The drawing under review shows one solid part. Ordinate dimensions are in mm from its lowest x, y, z. Coordinates: 2 decimals unless noted, no trailing zeros. Order: outer loops, then holes, each group sorted by start corner. A loop starts at its lowest first (then second) coordinate and runs counter-clockwise, first axis right, second up. Notation, with made-up numbers: (36.5, -12.5) -> (53.5, -12.5) arc R27 ccw to (53.5, 25.5) -> close; hole circle Ø5 at (33.5, -28). An arc over 180 degrees is marked (long way). Put each result on its own line as item: value.
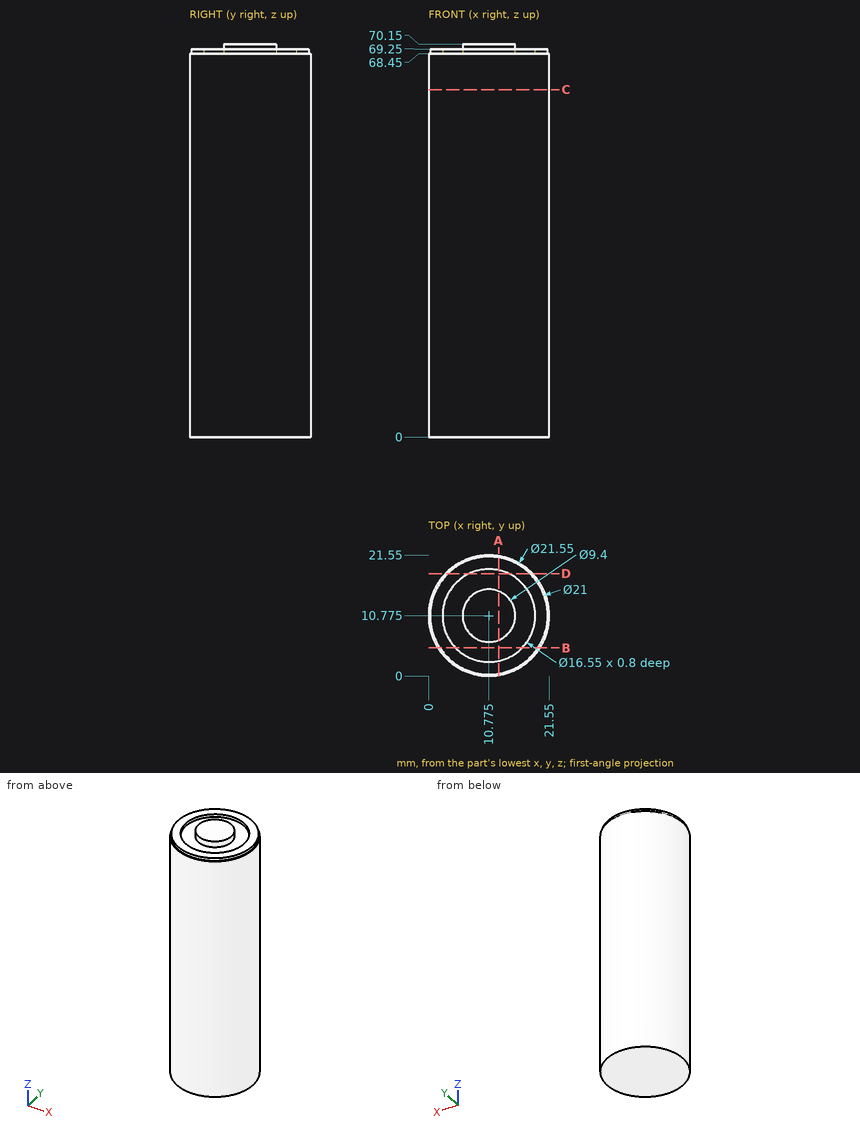
Item 1: Consider section B-B on y = 5. Write out the cut boundary in (x, z), and give its area (3 significant figures).
Answers below:
outline: (1.68, 0) -> (19.87, 0) -> (19.87, 68.45) -> (19.54, 68.45) -> (19.54, 69.25) -> (16.7, 69.25) -> (16.7, 68.45) -> (4.85, 68.45) -> (4.85, 69.25) -> (2.01, 69.25) -> (2.01, 68.45) -> (1.68, 68.45) -> close
area: 1,250 mm^2
Item 2: For pin 1 Ø12 at (x, z) = (6, 63) entering from +Y; pin 2 Ø3 at (x, z) = (4.5, 40) entering from +Y; pin 3 Ø12 at (y, z) = (19, 40) entering from -X; pin 4 Ø4 at (x, y) = (3, 18.5) entering from +Z, all flat-tipped, find the tip position at first contact; note any pin that passes through.
Answers below:
pin 1: y = 21.55
pin 2: y = 20.43
pin 3: x = 0.23
pin 4: z = 69.25
Item 3: Consider section D-D on y = 18.25. Write out the cut boundary in (x, z).
Answers below:
outline: (3.01, 0) -> (18.54, 0) -> (18.54, 68.45) -> (18.15, 68.45) -> (18.15, 69.25) -> (14.32, 69.25) -> (14.32, 68.45) -> (7.23, 68.45) -> (7.23, 69.25) -> (3.4, 69.25) -> (3.4, 68.45) -> (3.01, 68.45) -> close
Item 4: Consider section C-C on z = 62. Write out the cut boundary in (x, y) (3 decimals).
Answers below:
outline: circle Ø21.55 at (10.775, 10.775)
Item 5: Consider section A-A on x = 12.5. Write out the cut boundary in (y, z).
Answers below:
outline: (0.14, 0) -> (21.41, 0) -> (21.41, 68.45) -> (21.13, 68.45) -> (21.13, 69.25) -> (18.87, 69.25) -> (18.87, 68.45) -> (15.15, 68.45) -> (15.15, 70.15) -> (6.4, 70.15) -> (6.4, 68.45) -> (2.68, 68.45) -> (2.68, 69.25) -> (0.42, 69.25) -> (0.42, 68.45) -> (0.14, 68.45) -> close
Item 6: For line 1 (X direction, y = 11.25, z = 6.5); line 2 (Z direction, x = 2.5, y = 4.5), list the stretches that pass through material, from the lowest coordinate up. Write a range as from..to.
Answers below:
line 1: 0.01..21.54
line 2: 0..69.25
